The listing builds one solid part. Answer for the finished solid, in the listing's coordinates (mm). Round coordinates to 2 decimals unless told otherwise and drop trailing zeros. Loops run counter-clockwise (first coordinate to the right, second up) from the corner with the lowest first, then second, coordinate; pieces in that order, holes last. Notation, with made-up numbers: (42, -3) - (63, -3) arc R25 ccw to (63, 25) - close; hole circle Ø2 at (-0.75, 33). An arc over 180 degrees is marked (long way). Write item = value, one per line. Start each with the question number.
1) For a pull along Y with two mould halves and no side action, classify faces 1 (the flat face through (47, 4, 2)), 2 (the cylindrical face through (97.08, -0.86, 1.97)), 3 (the flat face through (48, 0, 0)) as released by +Y, released by -Y, zero draft, split by the parting line, or undercut.
2) Section A-A, the plane y = 1.25 is taken. Determine the outline of the cut face in (x, z), and give its area (3 significant figures).
3) Given pin 1 Ø5 at (x, z) = (58.5, 5) entering from +Y; pin 2 Ø2 at (x, y) = (66, -1) entering from +Z; pin 3 Ø4 at (y, z) = (3, 2) entering from -X, each flat-ended and moving along its own axis, determine where each tip first touches the part or whether it passes through.
4) Straight lines are drawn through the part: line 1 along X through (y, z) = (-0.25, 7); line 2 along Y through (x, z) = (0, 4.5); line 3 along X through (y, z) = (-0.5, 3). For each, find the intervals that lie inside material, in ascending order.
5) Section C-C, the plane x = 6.5 is taken. Determine the outline of the cut face in (y, z).
6) Section B-B, the plane z = 5 is taken. Determine the outline of the cut face in (x, y).
from build123d import *

# Parameters (mm, degrees)
SKETCH2_R               = 2.25
BOSS_EXTRUDE1_DEPTH     = 10
CUT_EXTRUDE_THIN1_START = -6
SKETCH3_R               = 104
SKETCH3_R_2             = 4
CUT_EXTRUDE_THIN1_DEPTH = 6


with BuildPart() as part:
    # Sketch2 → Boss-Extrude1 (new body)
    with BuildSketch(Plane.XY):
        with BuildLine():
            Line((0, 4), (95, 4))
            ThreePointArc((95, 4), (99, 0), (95, -4))
            Line((95, -4), (0, -4))
            ThreePointArc((0, -4), (-4, 0), (0, 4))
        make_face()
        Circle(SKETCH2_R, mode=Mode.SUBTRACT)
        with Locations((95, 0)):
            Circle(SKETCH2_R, mode=Mode.SUBTRACT)
    extrude(amount=BOSS_EXTRUDE1_DEPTH)

    # Sketch3 → Cut-Extrude-Thin1 (cut)
    with BuildSketch(Plane.XY.offset(10).offset(CUT_EXTRUDE_THIN1_START)):
        Circle(SKETCH3_R)
        Circle(SKETCH3_R_2, mode=Mode.SUBTRACT)
    extrude(amount=CUT_EXTRUDE_THIN1_DEPTH, mode=Mode.SUBTRACT)


solid = part.part
Geometry check:
q1.face_1 = released by +Y
q1.face_2 = undercut
q1.face_3 = zero draft
q2.outline = (-3.8, 0) - (-1.87, 0) - (-1.87, 10) - (-3.8, 10) - close; (1.87, 0) - (93.13, 0) - (93.13, 4) - (3.8, 4) - (3.8, 10) - (1.87, 10) - close; (96.87, 0) - (98.8, 0) - (98.8, 4) - (96.87, 4) - close
q2.area = 404 mm2
q3.pin_1 = 4
q3.pin_2 = 4
q3.pin_3 = -3.87
q4.line_1 = -3.99 to -2.24, 2.24 to 3.99
q4.line_2 = -4 to -2.25, 2.25 to 4
q4.line_3 = -3.97 to -2.19, 2.19 to 92.81, 97.19 to 98.97
q5.outline = (-4, 0) - (4, 0) - (4, 4) - (-4, 4) - close
q6.outline = circle Ø8 at (0, 0); hole circle Ø4.5 at (0, 0)
